Input: part model. Units: mm. Frame: model coordinates. A direction names the side the tool comes from. Round coordinates to 2 decimals unless told otherwise and drop trailing zeros. Order: outer loops, then holes, each group sorted by start corner. A loop starts at its lowest first (then second) coordinate and runs counter-clockwise, first axis right, second up. Notation, with made-up numbers: (13.25, 83.5) -> (56.25, 83.5) arc R24 cw to (56.25, 103.5) -> close; hole circle Ø4 at (-22.75, -39). An arc over 180 degrees is marked (long way). Use a Markdown table: item, result.
from build123d import *

# Parameters (mm, degrees)
F1_DEPTH = 25.4


with BuildPart() as f1:
    # F0 (on Front) → F1 (new body)
    with BuildSketch(Plane.XZ):
        Polygon((-7.659892, 41.999251), (-13.7416, 43.107137), (-15.429787, 33.990927), (-14.079237, 31.79628), (-12.728688, 26.731718), (-12.728688, 25.212349), (-12.728688, 21.329518), (-10.280816, 18.206371), (-7.832943, 15.083224), (-4.794206, 9.343385), (-1.586649, 5.460554), (3.646733, 4.110004), (7.023108, 4.110004), (10.905939, 7.824017), (14.95759, 15.083224), (18.321248, 18.31751), (19.346878, 19.303693), (20.528609, 26.731718), (20.528609, 30.10809), (22.554435, 33.990927), (20.528609, 43.107137), (15.543124, 41.999251), (10.735117, 36.532301), (4.320004, 38.220487), (-3.025021, 36.588258), align=None)
        Polygon((-7.832943, 15.083224), (-10.280816, 18.206371), (-15.09215, 1.577722), (3.646733, -31.510755), (22.047978, 0), (18.321248, 18.31751), (14.95759, 15.083224), (10.905939, 7.824017), (7.023108, 4.110004), (3.646733, 4.110004), (-1.586649, 5.460554), (-4.794206, 9.343385), align=None)
    extrude(amount=F1_DEPTH)


solid = f1.part
1) Cut plane C-C on x = 7. Return loops of the section in (y, z).
Results found:
| item | result |
|---|---|
| outline | (-25.4, -25.77) -> (0, -25.77) -> (0, 37.52) -> (-25.4, 37.52) -> close |
2) Line query: L1, parallel to X at y = -6.5, z = 0; L2, parallel to Z at x = -4.5, y = -16.5; L3, parallel to X at y = -1, z = 40. Output: solid intervals per line, ascending. Write a range as [from, to].
Results found:
| item | result |
|---|---|
| L1 | x = [-14.2, 22.05] |
| L2 | z = [-17.13, 38.31] |
| L3 | x = [-14.32, -5.95], [13.78, 21.22] |
3) Cut plane B-B on z = -27. Return loops of the section in (x, y), and give its area (3 significant figures).
Results found:
| item | result |
|---|---|
| outline | (1.09, -25.4) -> (6.28, -25.4) -> (6.28, 0) -> (1.09, 0) -> close |
| area | 132 mm² |
4) Set-up query: faces 1 (the flat face through (-12.653, -12.522, 10.008)), 2 (the flat face through (7.572, -12.522, 37.365)), 3 (the flat face through (20.21, -12.52, 9.03)). Return all of +Z, -Z, +X, -X, +Y, -Y with unobstructed straight access to the full face (end or side cutting, diameter ignored); none if empty.
Results found:
| item | result |
|---|---|
| face 1 | -X, +Y, -Y |
| face 2 | +Z, +Y, -Y |
| face 3 | +X, +Y, -Y |
5) Pin query (flat end, axial travel): pin 1 Ø2.5 at (y, z) = (-11.5, 24) entering from -X; pin 2 Ø12 at (x, y) = (15.5, -21) entering from +Z; pin 3 Ø1 at (x, y) = (-9, -10.5) entering from -Z. Return the tip coordinate at first contact, or that it passes through.
Results found:
| item | result |
|---|---|
| pin 1 | stops at x = -12.73 |
| pin 2 | stops at z = 43.11 |
| pin 3 | stops at z = -10.06 |
6) Cut plane A-A on y = -13.5. Return loops of the section in (x, z), and give its area (3 significant figures).
Results found:
| item | result |
|---|---|
| outline | (-15.43, 33.99) -> (-14.08, 31.8) -> (-12.73, 26.73) -> (-12.73, 21.33) -> (-10.28, 18.21) -> (-15.09, 1.58) -> (3.65, -31.51) -> (22.05, 0) -> (18.32, 18.32) -> (19.35, 19.3) -> (20.53, 26.73) -> (20.53, 30.11) -> (22.55, 33.99) -> (20.53, 43.11) -> (15.54, 42) -> (10.74, 36.53) -> (4.32, 38.22) -> (-3.03, 36.59) -> (-7.66, 42) -> (-13.74, 43.11) -> close |
| area | 1,910 mm² |
7) Pull-direction query (X, two-part tool) for faces 4 (the flat face through (-14.574, -12.522, 38.613)), 5 (the flat face through (21.556, -12.522, 38.485)), 6 (the flat face through (13.17, -12.52, 39.3)); classes: +X half, -X half, draft (parallel to the pull), parting line (faces both ways), or undercut.
Results found:
| item | result |
|---|---|
| face 4 | -X half |
| face 5 | +X half |
| face 6 | undercut |
